Autodesk Inventor part; units mm, degrees
ref_plane "YZ Plane" through (0, 0, 0) normal (1, 0, 0) x (0, 1, 0)
ref_plane "XZ Plane" through (0, 0, 0) normal (0, 1, 0) x (-1, 0, 0)
ref_plane "XY Plane" through (0, 0, 0) normal (0, 0, 1) x (1, 0, 0)
sketch "スケッチ1" plane through (0, 0, 0) normal (0, 0, 1) x (1, 0, 0)
  circle A0 centre (0, 0) radius 10
  dimension "d0" = 20
extrude "押し出し1" add sketch "スケッチ1" along normal blind 2.5
sketch "スケッチ2" plane through (0, 0, 2.5) normal (0, 0, 1) x (1, 0, 0)
  circle A0 centre (0, 0) radius 4.5
  dimension "d3" = 9
extrude "押し出し2" add sketch "スケッチ2" along normal blind 2.5
sketch "スケッチ3" plane through (0, 0, 0) normal (0, 0, -1) x (-1, 0, 0)
  circle A0 centre (0, 0) radius 10
  line L0 (0, 10) -> (0, -10)
  line L1 (-10, 0) -> (10, 0)
  point P0 (-5, 5)
  point P1 (5, 5)
  point P2 (5, -5)
  point P3 (-5, -5)
  dimension "d6" = 10
  dimension "d7" = 10
hole "穴1" at (5, 5, 0) at (-5, 5, 0) at (-5, -5, 0) at (5, -5, 0) direction (0, 0, 1) diameter 2.459 end through all
sketch "スケッチ4" plane through (0, 0, 5) normal (0, 0, -1) x (-1, 0, 0)
  point P0 (0, 0)
  point P1 (0, 0)
hole "穴2" at (0, 0, 5) direction (0, 0, -1) diameter 3 end through all counterbore diameter 6 counterbore depth 3.8
properties part number "サーボモータ25kgcmサーボホーン1" material "アルミニウム 6061"
Build history of the part. All positions in model axes, mm. A direction names the side the tool comes from. Coordinates: 2 decimals unless noted, no trailing zeros. Order: outer loops, then holes, each group sorted by start corner. A loop starts at its lowest first (then second) coordinate and runs counter-clockwise, first axis right, second up. Notation, with made-up numbers: M 64,52 L 84,52 A22 ccw 84,71 Z; hole C 66.25,28.5 d7. An arc over 180 degrees is marked long. One line per question, with ' | ' between items. Start each with the question number.
1. Tool access for faces 1 (the face through (0, 3, 3)), 2 (the face through (1, -3, 5)): list every direction of +Z, -Z, +X, -X, +Y, -Y with a clear straight run to the whole face (end or side of a thin tool).
2. Cut at A-A (x = 0). Write the cut outline in (y, z), plus the area to 3 significant figures.
3. Mould opens along Y. For faces 3 (the face through (-0.59, -4.46, 3.73)), 4 (the face through (5.748, 4.024, 1.268)), 5 (the face through (2, 0, 0)) say: +Y half, -Y half, draft (parallel to the pull), parting line (faces both ways), or undercut.
4. Cut at B-B (y = -0.75). Write the cut outline in (x, z), plus the area to 3 significant figures.
5. Flat gauge pins, fed straight in: P1, Ø3, axis at x = -5, y = -5, coming from the +Z side; P2, Ø1.5, axis at x = 5, y = 5, coming from the -Z side; P3, Ø1.5, axis at y = 2.5, z = 3, coming from the -X side. Where does each tip first touch, or does it go through?
6. Cut at C-C (z = 1.7). Write the cut outline in (x, y).
7. Cut at D-D (x = -4.25). Write the cut outline in (y, z).
8. Wall check: line 1 along Y through (x, z) = (0, 0.5); line 2 along X through (y, z) = (-5, 1.05); line 3 along Z through (x, y) = (6.25, 5.25). Give the ranges that are in metal, low to high. Write a range as [from, to].
The answers:
1) face 1: +Z | face 2: +Z, +X, -X, +Y, -Y
2) outline: M -10,0 L -1.5,0 L -1.5,1.2 L -3,1.2 L -3,5 L -4.5,5 L -4.5,2.5 L -10,2.5 Z; M 1.5,0 L 10,0 L 10,2.5 L 4.5,2.5 L 4.5,5 L 3,5 L 3,1.2 L 1.5,1.2 Z | area: 46.1 mm2
3) face 3: parting line | face 4: undercut | face 5: draft
4) outline: M -9.97,0 L -1.3,0 L -1.3,1.2 L -2.9,1.2 L -2.9,5 L -4.44,5 L -4.44,2.5 L -9.97,2.5 Z; M 1.3,0 L 9.97,0 L 9.97,2.5 L 4.44,2.5 L 4.44,5 L 2.9,5 L 2.9,1.2 L 1.3,1.2 Z | area: 46.9 mm2
5) P1: stops at z = 2.5 | P2: passes through | P3: stops at x = -9.81
6) outline: C 0,0 d20; hole C -5,-5 d2.46; hole C -5,5 d2.46; hole C 0,0 d6; hole C 5,-5 d2.46; hole C 5,5 d2.46
7) outline: M -9.05,0 L -5.97,0 L -5.97,2.5 L -9.05,2.5 Z; M -4.03,0 L 4.03,0 L 4.03,2.5 L 1.48,2.5 L 1.48,5 L -1.48,5 L -1.48,2.5 L -4.03,2.5 Z; M 5.97,0 L 9.05,0 L 9.05,2.5 L 5.97,2.5 Z
8) line 1: y = [-10, -1.5], [1.5, 10] | line 2: x = [-8.66, -6.23], [-3.77, 3.77], [6.23, 8.66] | line 3: z = [0, 2.5]
